Could you check a few things on this model? Use its own coordinates, in mm. A direction names the side the tool comes from. Give positions to 0.01 mm unless a question says otherwise; leave off trailing zeros. Order: outer loops, then holes, each group sorted by start corner. A loop starts at its lowest first (then second) coordinate and runs counter-clockwise, first axis right, second up. Notation, with made-up numbers: M 12,25.5 L 17,25.5 A12 cw 17,34.5 Z; hole C 11.5,-20 d6. An arc over 180 degrees is marked long. Use a Markdown table: item, result. Add a question column.
```python
from build123d import *

# Parameters (mm, degrees)
PAD_DEPTH    = 14
PAD001_DEPTH = 1
FILLET_R     = 4
FILLET001_R  = 1


with BuildPart() as part:
    # Sketch → Pad (new body, symmetric)
    with BuildSketch(Plane.XZ):
        with BuildLine():
            Line((-50.850763, 0), (50.850763, 0))
            ThreePointArc((50.850763, 0), (55.907413, 2.03282), (58.15, 7))
            Line((58.15, 7), (59, 27.3))
            Line((59, 27.3), (57, 27.3))
            Line((57, 27.3), (56.15, 7))
            ThreePointArc((50.936259, 2), (54.548152, 3.452014), (56.15, 7))
            Line((50.936259, 2), (0, 2))
            Line((0, 2), (-50.936259, 2))
            ThreePointArc((-56.15, 7), (-54.548152, 3.452014), (-50.936259, 2))
            Line((-56.15, 7), (-57, 27.3))
            Line((-57, 27.3), (-59, 27.3))
            Line((-59, 27.3), (-58.15, 7))
            ThreePointArc((-58.15, 7), (-55.907413, 2.03282), (-50.850763, 0))
        make_face()
    extrude(amount=PAD_DEPTH, both=True)

    # Sketch001 → Pad001 (join, symmetric)
    with BuildSketch(Plane.XZ):
        with BuildLine():
            Line((-58.3, 27.3), (-57.65, 34))
            ThreePointArc((-49.938031, 41), (-55.145585, 38.989037), (-57.65, 34))
            Line((-49.938031, 41), (0, 41))
            Line((0, 41), (49.938031, 41))
            ThreePointArc((57.65, 34), (55.145585, 38.989037), (49.938031, 41))
            Line((57.65, 34), (58.3, 27.3))
            Line((58.3, 27.3), (57.43949, 6.748988))
            ThreePointArc((51.444743, 1), (55.597689, 2.669523), (57.43949, 6.748988))
            Line((51.444743, 1), (-51.444743, 1))
            ThreePointArc((-57.43949, 6.748988), (-55.597689, 2.669523), (-51.444743, 1))
            Line((-58.3, 27.3), (-57.43949, 6.748988))
        make_face()
    extrude(amount=PAD001_DEPTH, both=True)

    # Fillet
    fillet_edges = [part.edges().sort_by_distance(p)[0] for p in [
        (-58, -14, 27.3),
        (58, -14, 27.3),
        (58, 14, 27.3),
        (-58, 14, 27.3),
    ]]
    fillet(fillet_edges, radius=FILLET_R)

    # Fillet001
    fillet001_edges = [part.edges().sort_by_distance(p)[0] for p in [
        (56.575, -1, 17.15),
        (56.575, 1, 17.15),
    ]]
    fillet(fillet001_edges, radius=FILLET001_R)


solid = part.part
```
1) For faces 5 (the face through (56.58, 7.92, 17.29)), 6 (the face through (1, -8, 2)), 7 (the face through (-55.09, -0.01, 39.04)), which set-ups out of +Z, -Z, +X, -X, +Y, -Y let a thin tool reach every point of the face, with its end or its side?
2) Please list where these lines run through material, in increasing order: line 1 (Z direction, x = -37, y = 3.25); line 2 (Y direction, x = -14.5, z = 19.5); line 3 (X direction, y = -2.75, z = 27). Write a range as from..to.
3) Suppose I cut it at B-B on y = 5.75. Please give me the cut outline in (x, z), and give its area (3 significant figures).
4) Suppose I cut it at A-A on x = -3. Please give me the cut outline in (y, z).
5) Suppose I cut it at C-C on z = 38. Please give me the cut outline in (x, y).
6) For pin 1 (1.5 mm diameter, centred on x = -22.5, z = 19, fed in from -Y); pin 2 (3.5 mm diameter, centred on x = -9.5, y = -8.5, fed in from +Z); pin 3 (5 mm diameter, centred on y = -6.5, z = 6, fed in from +X), each with a flat end and sliding along its axis, tell me the tip position at first contact or that it passes through.
7) We'd pull the mould along X, two halves only. Please class faces 1 (the face through (55.205, -0.014, 38.935)), 2 (the face through (56.58, -8.08, 17.29)), 3 (the face through (-58.5, -0.1, 27.3)), 4 (the face through (-56.57, -8.08, 17.01)): pulls with the +X half, pulls with the -X half, needs draft (parallel to the pull), parting line crosses it, or undercut.
Values found:
| question | item | result |
|---|---|---|
| 1 | face 5 | +Z, +Y |
| 1 | face 6 | +Z, -Y |
| 1 | face 7 | +Z, -X, +Y, -Y |
| 2 | line 1 | z = 0..2 |
| 2 | line 2 | y = -1..1 |
| 2 | line 3 | x = -58.99..-56.99, 56.99..58.99 |
| 3 | outline | M -59,27.3 L -58.15,7 A7.31 ccw -50.85,0 L 50.85,0 A7.31 ccw 58.15,7 L 59,27.3 L 57,27.3 L 56.15,7 A5.22 cw 50.94,2 L -50.94,2 A5.22 cw -56.15,7 L -57,27.3 Z |
| 3 | area | 323 mm^2 |
| 4 | outline | M -14,0 L 14,0 L 14,2 L 2,2 A1 cw 1,3 L 1,41 L -1,41 L -1,3 A1 cw -2,2 L -14,2 Z |
| 5 | outline | M -56.06,-1 L 56.06,-1 L 56.06,1 L -56.06,1 Z |
| 6 | pin 1 | stops at y = -1 |
| 6 | pin 2 | stops at z = 2 |
| 6 | pin 3 | stops at x = 58.21 |
| 7 | face 1 | pulls with the +X half |
| 7 | face 2 | undercut |
| 7 | face 3 | needs draft |
| 7 | face 4 | undercut |
